Verification items for this drawing (mm, ordinates from the low corner). A direction names the side the tool comes from. Round coordinates to 2 decimals unless told otherwise and drop trailing zeros. Loops run counter-clockwise (first coordinate to the right, second up) from the corner with the lowest first, then second, coordinate; pieces in that order, holes last. Notation, with made-up numbers: (33, 48) - (51, 48) arc R15 cw to (51, 58) - close; hole circle Ø4 at (-14.5, -21.5). An arc over 180 degrees is marked (long way). Answer in a Markdown table with one row per item. Add a question column.
(1) Cross-section at B-B on x = 8. Enter the section's corners in (y, z).
(2) Cross-section at C-C on z = 12.5. Enter the section's corners in (x, y), then the cut area to 3 significant figures.
(3) Mould release check, pull along Z, two halves, no side actions. Record for the marked faces 1, 2, 3 and 4: +Z half, -Z half, draft (parallel to the pull), parting line (faces both ways), or undercut.
(4) Access from +Z, -Z, +X, -X, +Y, -Y to the whole of each face (thin tool, end or side, straight path). Record for the marked faces 5 and 6.
(5) Thickness scan on line 1 along X through (y, z) = (13, 15.25); line 2 along Z through (x, y) = (60.5, 31.5); line 3 along Y through (x, z) = (8, 2). Record the ranges inside material, lowest first.
(6) Cross-section at D-D on y = 38. Enter the section's corners in (x, z).
(7) Gauge pin test, flat ends, axial feed: pin 1 (3 mm diameter, centred on x = 9, z = 14, fed in from +Y); pin 2 (3.5 mm diameter, centred on x = 58, y = 77.9, fed in from -Z); pin 3 (2.5 mm diameter, centred on x = 30.5, z = 20, fed in from +Y); pin 4 (10.5 mm diameter, centred on x = 33, y = 38, fed in from +Z). Record the tip position at first contact, or that the pin passes through.
(8) Cross-section at A-A on y = 77.9. Enter the section's corners in (x, z).
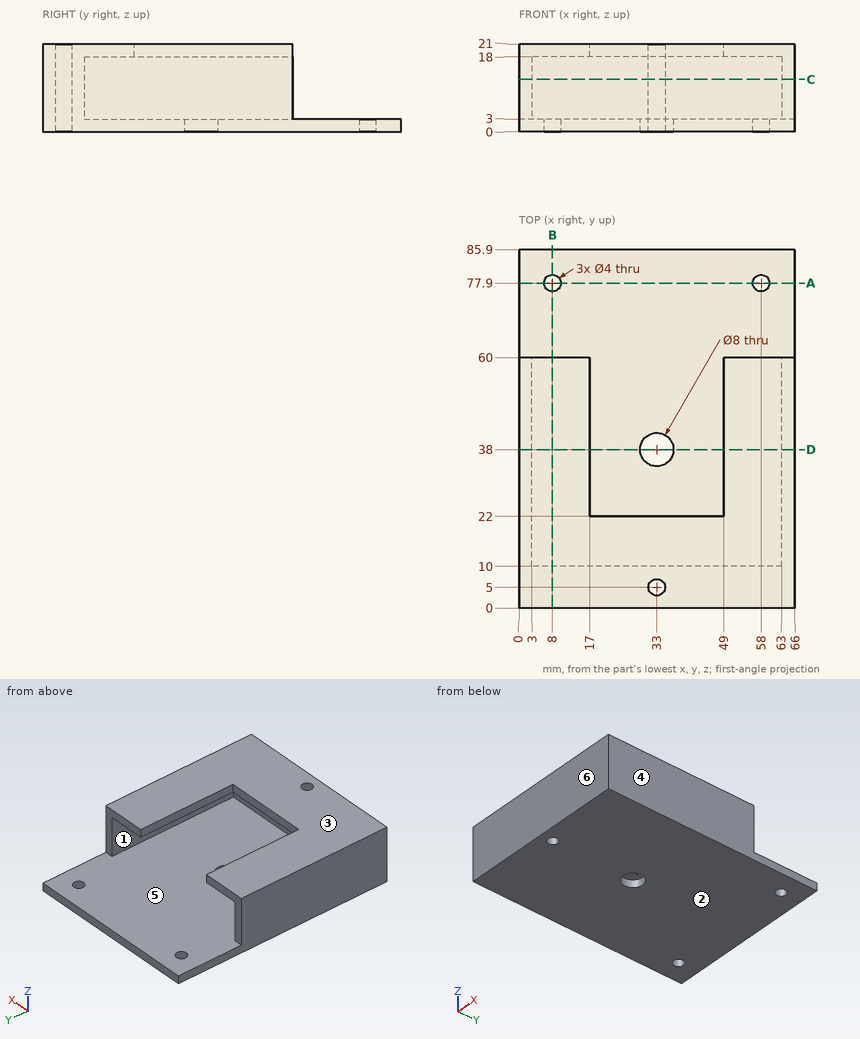
Answers:
| question | item | result |
|---|---|---|
| 1 | outline | (0, 0) - (75.9, 0) - (75.9, 3) - (10, 3) - (10, 18) - (60, 18) - (60, 21) - (0, 21) - close; (79.9, 0) - (85.9, 0) - (85.9, 3) - (79.9, 3) - close |
| 2 | outline | (0, 0) - (66, 0) - (66, 60) - (63, 60) - (63, 10) - (3, 10) - (3, 60) - (0, 60) - close; hole circle Ø4 at (33, 5) |
| 2 | area | 947 mm^2 |
| 3 | face 1 | undercut |
| 3 | face 2 | -Z half |
| 3 | face 3 | +Z half |
| 3 | face 4 | draft |
| 4 | face 5 | +Y |
| 4 | face 6 | +Z, -Z, +X, -X, -Y |
| 5 | line 1 | x = 0 to 3, 63 to 66 |
| 5 | line 2 | z = 0 to 3, 18 to 21 |
| 5 | line 3 | y = 0 to 75.9, 79.9 to 85.9 |
| 6 | outline | (0, 0) - (29, 0) - (29, 3) - (3, 3) - (3, 18) - (17, 18) - (17, 21) - (0, 21) - close; (37, 0) - (66, 0) - (66, 21) - (49, 21) - (49, 18) - (63, 18) - (63, 3) - (37, 3) - close |
| 7 | pin 1 | stops at y = 10 |
| 7 | pin 2 | passes through |
| 7 | pin 3 | stops at y = 22 |
| 7 | pin 4 | stops at z = 3 |
| 8 | outline | (0, 0) - (6, 0) - (6, 3) - (0, 3) - close; (10, 0) - (56, 0) - (56, 3) - (10, 3) - close; (60, 0) - (66, 0) - (66, 3) - (60, 3) - close |
